from build123d import *

# Parameters (mm, degrees)
F1_DEPTH = 16.256
F2_W     = 51.8002919853
F2_H     = 14.5590286702
F3_DEPTH = 100.33
F5_DEPTH = 39.116
F6_DEPTH = 25.4
F7_W     = 13.6753991246
F7_H     = 28.8449618965
F8_DEPTH = 31.242


with BuildPart() as f1:
    # F0 (on Top) → F1 (new body)
    with BuildSketch(Plane.XY):
        with BuildLine():
            Line((-25.9001459926, -27.6933182031), (25.9001459926, -27.6933182031))
            Line((25.9001459926, -27.6933182031), (25.9001459926, 27.6933182031))
            ThreePointArc((25.9001459926, 27.6933182031), (0, 53.5934641957), (-25.9001459926, 27.6933182031))
            Line((-25.9001459926, 27.6933182031), (-25.9001459926, -27.6933182031))
        make_face()
    extrude(amount=F1_DEPTH)

    # F2 (on face) → F3 (join)
    with BuildSketch(Plane.XY.offset(16.256)):
        with Locations((0, -20.413803868)):
            Rectangle(F2_W, F2_H)
    extrude(amount=F3_DEPTH)

    # F4 (on face) → F5 (cut)
    with BuildSketch(Plane(origin=(0, -13.1342895329, 0), x_dir=(-1, 0, 0), z_dir=(0, 1, 0))):
        with BuildLine():
            Line((10.1979328319, 54.3813481927), (10.1979328319, 116.5178194642))
            Line((10.1979328319, 116.5178194642), (-10.1979328319, 116.5178194642))
            Line((-10.1979328319, 116.5178194642), (-10.1979328319, 54.3813481927))
            ThreePointArc((-10.1979328319, 54.3813481927), (0, 44.1834153607), (10.1979328319, 54.3813481927))
        make_face()
    extrude(amount=-F5_DEPTH, mode=Mode.SUBTRACT)

    # F6 (cut): a face of the model
    f6_faces = [f1.faces().sort_by_distance(p)[0] for p in [
        (0, -20.413803868, 116.5178194642),
    ]]
    extrude(f6_faces, amount=-F6_DEPTH, mode=Mode.SUBTRACT)

    # F7 (on face) → F8 (cut)
    with BuildSketch(Plane.XZ.offset(27.6933182031)):
        with Locations((-19.0624464303, 14.4224809483)):
            Rectangle(F7_W, F7_H)
    extrude(amount=-F8_DEPTH, mode=Mode.SUBTRACT)


solid = f1.part
Geometry: final body of the model. Coordinates: model frame, mm. A direction names the side the tool comes from. Give positions to 0.01 mm unless a question says otherwise; leave off trailing zeros. Order: outer loops, then holes, each group sorted by start corner. A loop starts at its lowest first (then second) coordinate and runs counter-clockwise, first axis right, second up. Notation, with made-up numbers: (69.25, -16) -> (115.25, -16) arc R11 cw to (115.25, 1) -> close; hole circle Ø4 at (-2.5, 85). An arc over 180 degrees is marked (long way). Answer as a JSON object with one key per item and string values.
Q1. Access query for faces 1 (the flat face through (-12.225, -16, 11)), 2 (the flat face through (-19, 3.549, 8)), 3 (the flat face through (11, -13.134, 66)), 4 (the flat face through (10.198, -20, 85)). Directions: +Z, -Z, +X, -X, +Y, -Y. A direction counts if a zero-diameter tool reaches every point of the face in a straight line with its end or side. Return the directions, or none.
Entries:
{"face 1": "-Z, -X, -Y", "face 2": "+Z, -Z, -X, -Y", "face 3": "+Z, +X, -X, +Y", "face 4": "+Z, +Y, -Y"}
Q2. Section B-B (y = -19.5). Output: boundary loops of the cut face in (x, z).
Entries:
{"outline": "(-25.9, 28.84) -> (-12.22, 28.84) -> (-12.22, 0) -> (25.9, 0) -> (25.9, 116.59) -> (10.2, 116.59) -> (10.2, 54.38) arc R10.2 cw to (-10.2, 54.38) -> (-10.2, 116.59) -> (-25.9, 116.59) -> close"}
Q3. Section A-A (z = 73). Output: boundary loops of the cut face in (x, y), plus the area to 3 significant figures.
Entries:
{"outline": "(-25.9, -27.69) -> (-10.2, -27.69) -> (-10.2, -13.13) -> (-25.9, -13.13) -> close; (10.2, -27.69) -> (25.9, -27.69) -> (25.9, -13.13) -> (10.2, -13.13) -> close", "area": "457 mm^2"}
Q4. Draft query along X for faces 5 (the cylindrical face through (0.224, -20.312, 44.186)), 6 (the flat face through (-10.198, -20, 85)), 7 (the cylindrical face through (0.57, 53.587, 8.014)), 8 (the flat face through (0, 21, 16.256)). Return one class per face: released by +X, released by -X, zero draft, split by the parting line, or undercut.
Entries:
{"face 5": "undercut", "face 6": "undercut", "face 7": "split by the parting line", "face 8": "zero draft"}
Q5. Section C-C (z = 11.5). Output: boundary loops of the cut face in (x, y).
Entries:
{"outline": "(-25.9, 3.55) -> (-12.22, 3.55) -> (-12.22, -27.69) -> (25.9, -27.69) -> (25.9, 27.69) arc R25.9 ccw to (-25.9, 27.69) -> close"}
Q6. First-contact query: pin 1 (7 mm diameter, centred on x = -16.5, y = -20, fed in from -Z); pin 2 (8 mm diameter, centred on x = -18.5, z = 76, fed in from +Y); pin 3 (2 mm diameter, centred on x = 2.5, y = -9.5, fed in from +Z). Flat tips, straight axial feed; report the tip coordinate or a pass-through.
Entries:
{"pin 1": "stops at z = 28.84", "pin 2": "stops at y = -13.13", "pin 3": "stops at z = 16.26"}
Q7. Section D-D (x = 0). Output: boundary loops of the cut face in (y, z), plus the area to 3 significant figures.
Entries:
{"outline": "(-27.69, 0) -> (53.59, 0) -> (53.59, 16.26) -> (-13.13, 16.26) -> (-13.13, 44.18) -> (-27.69, 44.18) -> close", "area": "1,730 mm^2"}
Q8. Material intervals for probe 1 along Y at (x, z) = (22.5, 25.5); probe 2 along Z at (x, y) = (4, 20); probe 3 along Z at (x, y) = (-18, -16), sorted ascending.
Entries:
{"probe 1": "y = -27.69 to -13.13", "probe 2": "z = 0 to 16.26", "probe 3": "z = 28.84 to 116.59"}
